Read the model definition and answer for the solid it produces. Units are mm, in the model's axes. Coordinates: 2 decimals unless noted, no trailing zeros. Write each loop counter-clockwise with the first axis right and the second up, starting at its lowest first coordinate (ties: lowest second). Pieces come first, ordered by that corner, then holes. Notation, with made-up numbers: (47.25, 58) - (85.25, 58) arc R27 cw to (85.25, 88) - close; hole circle Ø5 at (-38.5, 33). An arc over 180 degrees is marked (long way). Return JSON: item names as keys, results as strings.
Autodesk Inventor part; units mm, degrees
ref_plane "YZ Plane" through (0, 0, 0) normal (1, 0, 0) x (0, 1, 0)
ref_plane "XZ Plane" through (0, 0, 0) normal (0, 1, 0) x (-1, 0, 0)
ref_plane "XY Plane" through (0, 0, 0) normal (0, 0, 1) x (1, 0, 0)
sketch "Sketch1" plane through (0, 0, 0) normal (0, 1, 0) x (-1, 0, 0)
  line L0 (22.4826, 148.6372) -> (-167.5174, 148.6372)
  line L1 (-167.5174, 148.6372) -> (-167.5174, 3.6372)
  line L2 (-167.5174, 3.6372) -> (22.4826, 3.6372)
  line L3 (22.4826, 3.6372) -> (22.4826, 148.6372)
  line L4 (-167.5174, 88.6372) -> (-172.5174, 88.6372)
  line L5 (-172.5174, 88.6372) -> (-172.5174, 63.6372)
  line L6 (-172.5174, 63.6372) -> (-167.5174, 63.6372)
  line L7 (-167.5174, 63.6372) -> (-167.5174, 88.6372)
  line L8 (-167.5174, 43.6372) -> (-172.5174, 43.6372)
  line L9 (-172.5174, 43.6372) -> (-172.5174, 18.6372)
  line L10 (-172.5174, 18.6372) -> (-167.5174, 18.6372)
  line L11 (-167.5174, 18.6372) -> (-167.5174, 43.6372)
  line L12 (-72.5174, 148.6372) -> (-72.5174, 3.6372) construction
  line L13 (22.4826, 88.6372) -> (27.4826, 88.6372)
  line L14 (27.4826, 88.6372) -> (27.4826, 63.6372)
  line L15 (27.4826, 63.6372) -> (22.4826, 63.6372)
  line L16 (22.4826, 43.6372) -> (27.4826, 43.6372)
  line L17 (27.4826, 43.6372) -> (27.4826, 18.6372)
  line L18 (27.4826, 18.6372) -> (22.4826, 18.6372)
  point P0 (0, 0)
  dimension "d0" = 190
  dimension "d1" = 145
  dimension "d2" = 5
  dimension "d3" = 25
  dimension "d4" = 5
  dimension "d5" = 25
  dimension "d6" = 20
  dimension "d7" = 15
extrude "Extrusion1" add sketch "Sketch1" along normal blind 5
sketch "Sketch2" plane through (0, 5, 0) normal (0, 1, 0) x (1, 0, 0)
  line L0 (-27.4826, -43.6372) -> (-22.4826, -43.6372)
  line L1 (-22.4826, -43.6372) -> (-22.4826, -63.6372)
  line L2 (-22.4826, -63.6372) -> (-27.4826, -63.6372)
  line L3 (-27.4826, -63.6372) -> (-27.4826, -88.6372)
  line L4 (-27.4826, -88.6372) -> (-22.4826, -88.6372)
  line L5 (-22.4826, -88.6372) -> (-22.4826, -148.6372)
  line L6 (-22.4826, -148.6372) -> (167.5174, -148.6372)
  line L7 (167.5174, -148.6372) -> (167.5174, -88.6372)
  line L8 (167.5174, -88.6372) -> (172.5174, -88.6372)
  line L9 (172.5174, -88.6372) -> (172.5174, -63.6372)
  line L10 (172.5174, -63.6372) -> (167.5174, -63.6372)
  line L11 (167.5174, -63.6372) -> (167.5174, -43.6372)
  line L12 (167.5174, -43.6372) -> (172.5174, -43.6372)
  line L13 (172.5174, -43.6372) -> (172.5174, -18.6372)
  line L14 (172.5174, -18.6372) -> (167.5174, -18.6372)
  line L15 (167.5174, -18.6372) -> (167.5174, -3.6372)
  line L16 (167.5174, -3.6372) -> (-22.4826, -3.6372)
  line L17 (-22.4826, -3.6372) -> (-22.4826, -18.6372)
  line L18 (-22.4826, -18.6372) -> (-27.4826, -18.6372)
  line L19 (-27.4826, -18.6372) -> (-27.4826, -43.6372)
  line L20 (80.5174, -108.6372) -> (122.5174, -108.6372)
  line L21 (122.5174, -108.6372) -> (122.5174, -54.6372)
  line L22 (122.5174, -54.6372) -> (80.5174, -54.6372)
  line L23 (80.5174, -54.6372) -> (80.5174, -108.6372)
  point P0 (0, 0)
  dimension "d10" = 42
  dimension "d11" = 54
  dimension "d12" = 45
  dimension "d13" = 40
extrude "Extrusion2" cut sketch "Sketch2" against normal blind 5 contours L23 L22 L21 L20
properties part number "Top 2"
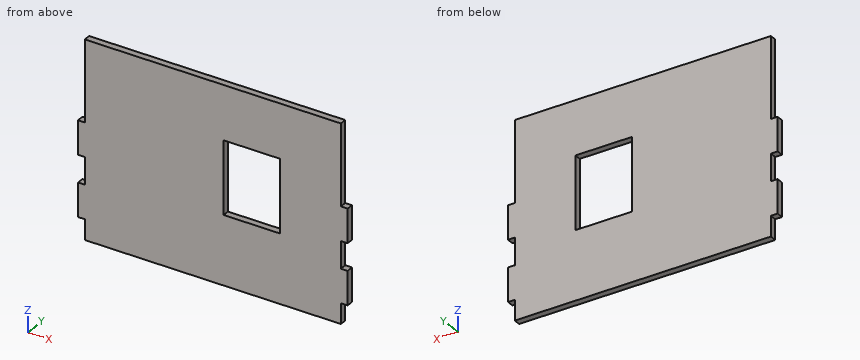
(1) A cutting plane is placed at C-C (y = 2). Determine the outline of the cut face in (x, z), and give its area (3 significant figures).
Answer:
{"outline": "(-27.48, 18.64) - (-22.48, 18.64) - (-22.48, 3.64) - (167.52, 3.64) - (167.52, 18.64) - (172.52, 18.64) - (172.52, 43.64) - (167.52, 43.64) - (167.52, 63.64) - (172.52, 63.64) - (172.52, 88.64) - (167.52, 88.64) - (167.52, 148.64) - (-22.48, 148.64) - (-22.48, 88.64) - (-27.48, 88.64) - (-27.48, 63.64) - (-22.48, 63.64) - (-22.48, 43.64) - (-27.48, 43.64) - close; hole (80.52, 54.64) - (122.52, 54.64) - (122.52, 108.64) - (80.52, 108.64) - close", "area": "25,800 mm²"}
(2) A cutting plane is placed at B-B (x = 110). Determine the outline of the cut face in (y, z), and give its area (3 significant figures).
Answer:
{"outline": "(0, 3.64) - (5, 3.64) - (5, 54.64) - (0, 54.64) - close; (0, 108.64) - (5, 108.64) - (5, 148.64) - (0, 148.64) - close", "area": "455 mm²"}
(3) Flat-ended cylindrical pins translate along their axes: P1, Ø2.5, axis at x = 169, y = 2.5, coming from the +Z side; P2, Ø1.5, axis at y = 2.5, z = 13, coming from the -X side; P3, Ø2.5, axis at y = 2, z = 109.5, coming from the +X side. Find the tip coordinate at first contact, or state that the pin passes through.
Answer:
{"P1": "z = 88.64", "P2": "x = -22.48", "P3": "x = 167.52"}
(4) Straight lines are drawn through the part: line 1 (Z direction, x = 104, y = 2.75); line 2 (X direction, y = 4.15, z = 60.5); line 3 (X direction, y = 0.4, z = 10.5). For each, find the intervals that lie inside material, in ascending order. Write a range as from..to.
Answer:
{"line 1": "3.64..54.64, 108.64..148.64", "line 2": "-22.48..80.52, 122.52..167.52", "line 3": "-22.48..167.52"}
(5) A cutting plane is placed at A-A (z = 61.5). Determine the outline of the cut face in (x, y), and give its area (3 significant figures).
Answer:
{"outline": "(-22.48, 0) - (80.52, 0) - (80.52, 5) - (-22.48, 5) - close; (122.52, 0) - (167.52, 0) - (167.52, 5) - (122.52, 5) - close", "area": "740 mm²"}
(6) A cutting plane is placed at D-D (z = 137). Determine the outline of the cut face in (x, y), and give its area (3 significant figures).
Answer:
{"outline": "(-22.48, 0) - (167.52, 0) - (167.52, 5) - (-22.48, 5) - close", "area": "950 mm²"}
